Can you work these out from the model? Positions are in its coordinate system, mm. A direction names the side the tool comes from. Give positions to 0.01 mm unless a question says otherwise; leave off trailing zeros. Order: outer loops, then holes, each group sorted by start corner. A loop starts at its lowest first (then second) coordinate and runs counter-clockwise, first axis right, second up. Notation, with made-up numbers: (-25, -39) - (23, -39) arc R30 ccw to (23, -10) - close; hole circle Ø1 at (-25.75, 42.5). An arc over 180 degrees is marked (long way). One line per question, with ' | ' between items.
```python
from build123d import *

# Parameters (mm, degrees)
SALIENTE_EXTRUIR1_DEPTH = 14
CROQUIS2_R              = 2.6
CORTAR_EXTRUIR1_DEPTH   = 14
CORTAR_EXTRUIR2_DEPTH   = 15
CROQUIS4_R              = 2
CORTAR_EXTRUIR3_DEPTH   = 31


with BuildPart() as part:
    # Croquis1 → Saliente-Extruir1 (new body)
    with BuildSketch(Plane.XY):
        Polygon((-9, 6), (-9, 32.8), (9, 32.8), (9, 6), (21, 6), (21, 0), (-21, 0), (-21, 6), align=None)
    extrude(amount=SALIENTE_EXTRUIR1_DEPTH)

    # Croquis2 → Cortar-Extruir1 (cut)
    with BuildSketch(Plane(origin=(0, 6, 0), x_dir=(1, 0, 0), z_dir=(0, 1, 0))):
        with Locations((-16.05, -7)):
            Circle(CROQUIS2_R)
        with Locations((16.05, -7)):
            Circle(CROQUIS2_R)
    extrude(amount=-CORTAR_EXTRUIR1_DEPTH, mode=Mode.SUBTRACT)

    # Croquis3 → Cortar-Extruir2 (cut, through all)
    with BuildSketch(Plane.XY.offset(14)):
        with BuildLine():
            Line((-1, 23.872983346), (-1, 32.8))
            Line((-1, 32.8), (1, 32.8))
            Line((1, 32.8), (1, 23.872983346))
            ThreePointArc((1, 23.872983346), (0, 16), (-1, 23.872983346))
        make_face()
    extrude(amount=-CORTAR_EXTRUIR2_DEPTH, mode=Mode.SUBTRACT)

    # Croquis4 → Cortar-Extruir3 (cut, through all)
    with BuildSketch(Plane.ZY.offset(9)):
        with Locations((7, 27.8)):
            Circle(CROQUIS4_R)
    extrude(amount=-CORTAR_EXTRUIR3_DEPTH, mode=Mode.SUBTRACT)


solid = part.part
```
(1) If we mould it in two halves opening along Z, with no side actions, what happens to faces 1 (the face through (4.944, 29.783, 6.74)), 2 (the face through (0, 9, 14)), 3 (the face through (-21, 3, 7))? For each: released by +Z, released by -Z, zero draft, split by the parting line, or undercut.
Answer below:
face 1: undercut | face 2: released by +Z | face 3: zero draft
(2) On a 3-axis mill with a long thin cutter (end or side, diameter ignored), from which of +Z, -Z, +X, -X, +Y, -Y can I reach the whole of each face in a straight line? I mean faces 4 (the face through (-1, 29, 9)), 5 (the face through (0, 9, 0)), 6 (the face through (-9, 19, 7)), 7 (the face through (9, 20, 7)). Say none if no direction works.
Answer below:
face 4: +Z, -Z, +Y | face 5: -Z, +X, -X, +Y, -Y | face 6: +Z, -Z, -X, +Y | face 7: +Z, -Z, +X, +Y
(3) Imagine slicing it at A-A (y = 27.8). List the corners of the cut face in (x, z) for me, and give its area (3 significant figures).
Answer below:
outline: (-9, 0) - (-1, 0) - (-1, 5) - (-9, 5) - close; (-9, 9) - (-1, 9) - (-1, 14) - (-9, 14) - close; (1, 0) - (9, 0) - (9, 5) - (1, 5) - close; (1, 9) - (9, 9) - (9, 14) - (1, 14) - close | area: 160 mm^2
(4) Imagine slicing it at C-C (x = 16.05). List the corners of the cut face in (y, z) for me, and give its area (3 significant figures).
Answer below:
outline: (0, 0) - (6, 0) - (6, 4.4) - (0, 4.4) - close; (0, 9.6) - (6, 9.6) - (6, 14) - (0, 14) - close | area: 52.8 mm^2
(5) Will these pins go through, and if not, where does the flat tip stop? pin 1 (3.5 mm diameter, centred on y = 27.8, z = 7, fed in from -X); pin 2 (6 mm diameter, centred on x = 16.05, z = 7, fed in from -Y); pin 3 (4 mm diameter, centred on y = 19, z = 9, fed in from -X); pin 4 (7 mm diameter, centred on y = 26, z = 8, fed in from +X).
Answer below:
pin 1: through | pin 2: y = 0 | pin 3: x = -9 | pin 4: x = 9
(6) If I drill on line 1 (X direction, y = 2.05, z = 7); line 2 (Z direction, x = -16, y = 2); line 3 (Y direction, x = -6.75, z = 7), over which ranges is the centre line in solid material (lowest first)?
Answer below:
line 1: -21 to -18.65, -13.45 to 13.45, 18.65 to 21 | line 2: 0 to 4.4, 9.6 to 14 | line 3: 0 to 25.8, 29.8 to 32.8
(7) Imagine slicing it at B-B (z = 7). List the corners of the cut face in (x, y) for me, and give its area (3 significant figures).
Answer below:
outline: (-21, 0) - (-18.65, 0) - (-18.65, 6) - (-21, 6) - close; (-13.45, 0) - (13.45, 0) - (13.45, 6) - (9, 6) - (9, 25.8) - (1, 25.8) - (1, 23.87) arc R4 cw (long way) to (-1, 23.87) - (-1, 25.8) - (-9, 25.8) - (-9, 6) - (-13.45, 6) - close; (-9, 29.8) - (-1, 29.8) - (-1, 32.8) - (-9, 32.8) - close; (1, 29.8) - (9, 29.8) - (9, 32.8) - (1, 32.8) - close; (18.65, 0) - (21, 0) - (21, 6) - (18.65, 6) - close | area: 540 mm^2
(8) Imagine slicing it at D-D (z = 2). List the corners of the cut face in (x, y) for me.
Answer below:
outline: (-21, 0) - (21, 0) - (21, 6) - (9, 6) - (9, 32.8) - (1, 32.8) - (1, 23.87) arc R4 cw (long way) to (-1, 23.87) - (-1, 32.8) - (-9, 32.8) - (-9, 6) - (-21, 6) - close
